from build123d import *

# Parameters (mm, degrees)
SKETCH_W        = 54.3
SKETCH_H        = 38
PAD_DEPTH       = 2
SKETCH001_W     = 54.3
SKETCH001_H     = 2
PAD001_DEPTH    = 22
SKETCH002_R     = 2.95
PAD002_DEPTH    = 5
SKETCH003_W     = 6.85
SKETCH003_H     = 15
PAD003_DEPTH    = 22
SKETCH004_R     = 1.5
POCKET_DEPTH    = 15
SKETCH005_W     = 6.85
SKETCH005_H     = 15
PAD004_DEPTH    = 22
SKETCH006_R     = 1.5
POCKET001_DEPTH = 15
CHAMFER_SIZE    = 0.5


with BuildPart() as part:
    # Sketch → Pad (new body)
    with BuildSketch(Plane.XY):
        with Locations((27.15, 21)):
            Rectangle(SKETCH_W, SKETCH_H)
    extrude(amount=PAD_DEPTH)

    # Sketch001 → Pad001 (join)
    with BuildSketch(Plane.XY):
        with Locations((27.15, 1)):
            Rectangle(SKETCH001_W, SKETCH001_H)
    extrude(amount=PAD001_DEPTH)

    # Sketch002 → Pad002 (join)
    with BuildSketch(Plane.XZ):
        with Locations((37.25, 12)):
            Circle(SKETCH002_R)
    extrude(amount=PAD002_DEPTH)

    # Sketch003 → Pad003 (join)
    with BuildSketch(Plane.XY):
        with Locations((3.425, 20.3)):
            Rectangle(SKETCH003_W, SKETCH003_H)
    extrude(amount=PAD003_DEPTH)

    # Sketch004 (on Face14 of Pad003) → Pocket (cut)
    with BuildSketch(Plane(origin=(0, 27.8, 0), x_dir=(-1, 0, 0), z_dir=(0, 1, 0))):
        with Locations((-3, 17)):
            Circle(SKETCH004_R)
        with Locations((-3, 7)):
            Circle(SKETCH004_R)
    extrude(amount=-POCKET_DEPTH, mode=Mode.SUBTRACT)

    # Sketch005 → Pad004 (join)
    with BuildSketch(Plane.XY):
        with Locations((50.875, 20.3)):
            Rectangle(SKETCH005_W, SKETCH005_H)
    extrude(amount=PAD004_DEPTH)

    # Sketch006 (on Face13 of Pad004) → Pocket001 (cut)
    with BuildSketch(Plane(origin=(0, 27.8, 0), x_dir=(-1, 0, 0), z_dir=(0, 1, 0))):
        with Locations((-51.3, 17)):
            Circle(SKETCH006_R)
        with Locations((-51.3, 7)):
            Circle(SKETCH006_R)
    extrude(amount=-POCKET001_DEPTH, mode=Mode.SUBTRACT)

    # Chamfer
    chamfer_edges = [part.edges().sort_by_distance(p)[0] for p in [
        (34.3, -5, 12),
    ]]
    chamfer(chamfer_edges, length=CHAMFER_SIZE)


solid = part.part
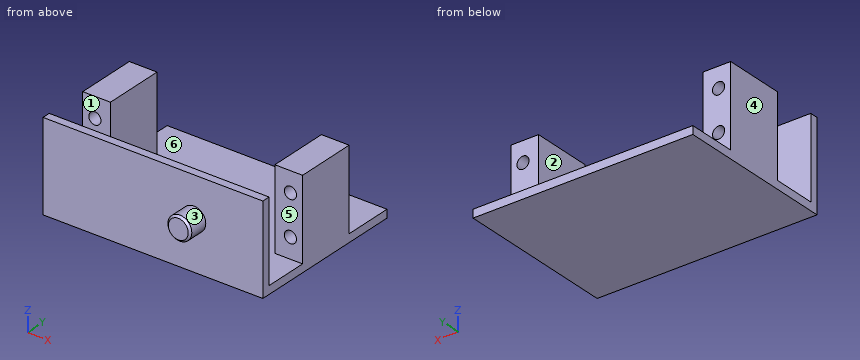
Could you check a few things on this model? Use its own coordinates, in mm. Face numbers are marked on the shaded views. A direction names the side the tool comes from. Round coordinates to 2 decimals unless told otherwise and drop trailing zeros. Write each loop counter-clockwise with the first axis right and the second up, starting at its lowest first coordinate (ties: lowest second). Pieces come first, ordered by that corner, then holes. Notation, with made-up numbers: (36.25, -40) - (45.25, -40) arc R26 ccw to (45.25, -24) - close; hole circle Ø9 at (18, 10.5). An arc over 180 degrees is marked (long way). Use a Markdown table: item, result.
Q1. I want a section at A-A (x = 51.3). List the corners of the cut face in (y, z) for me, plus the area to 3 significant figures.
Output values:
| item | result |
|---|---|
| outline | (0, 0) - (40, 0) - (40, 2) - (27.8, 2) - (27.8, 5.5) - (12.8, 5.5) - (12.8, 2) - (2, 2) - (2, 22) - (0, 22) - close; (12.8, 8.5) - (27.8, 8.5) - (27.8, 15.5) - (12.8, 15.5) - close; (12.8, 18.5) - (27.8, 18.5) - (27.8, 22) - (12.8, 22) - close |
| area | 330 mm2 |
Q2. For pin 1 (5 mm diameter, centred on x = 3, z = 7, fed in from -Y); pin 2 (5 mm diameter, centred on x = 46, y = 34, fed in from +Z); pin 3 (3.5 mm diameter, centred on x = 3, z = 17, fed in from +Y), each with a flat end and sliding along its axis, tell me the tip position at first contact or that it passes through.
Output values:
| item | result |
|---|---|
| pin 1 | y = 0 |
| pin 2 | z = 2 |
| pin 3 | y = 27.8 |
Q3. I want a section at B-B (z = 7). List the corners of the cut face in (x, y) for me.
Output values:
| item | result |
|---|---|
| outline | (0, 0) - (54.3, 0) - (54.3, 2) - (0, 2) - close; (0, 12.8) - (1.5, 12.8) - (1.5, 27.8) - (0, 27.8) - close; (4.5, 12.8) - (6.85, 12.8) - (6.85, 27.8) - (4.5, 27.8) - close; (47.45, 12.8) - (49.8, 12.8) - (49.8, 27.8) - (47.45, 27.8) - close; (52.8, 12.8) - (54.3, 12.8) - (54.3, 27.8) - (52.8, 27.8) - close |
Q4. Please list where these lines run through material, in increasing order: L1, parallel to Z at x = 3, y = 18; L2, parallel to X at y = 14.5, z = 9; L3, parallel to Y at x = 47.5, z = 14.5.
Output values:
| item | result |
|---|---|
| L1 | 0 to 5.5, 8.5 to 15.5, 18.5 to 22 |
| L2 | 0 to 6.85, 47.45 to 54.3 |
| L3 | 0 to 2, 12.8 to 27.8 |
Q5. For the marked faces 1, 2 and 3, which set-ups out of +Z, -Z, +X, -X, +Y, -Y let a thin tool reach every point of the face, with its end or its side?
Output values:
| item | result |
|---|---|
| face 1 | +Z, +X, -X |
| face 2 | +Z, +Y |
| face 3 | -Y |
Q6. I want a section at D-D (x = 33). List the corners of the cut face in (y, z) for me.
Output values:
| item | result |
|---|---|
| outline | (0, 0) - (40, 0) - (40, 2) - (2, 2) - (2, 22) - (0, 22) - close |
Q7. I want a section at C-C (z = 19.25). List the corners of the cut face in (x, y) for me.
Output values:
| item | result |
|---|---|
| outline | (0, 0) - (54.3, 0) - (54.3, 2) - (0, 2) - close; (0, 12.8) - (6.85, 12.8) - (6.85, 27.8) - (0, 27.8) - close; (47.45, 12.8) - (54.3, 12.8) - (54.3, 27.8) - (47.45, 27.8) - close |
Q8. Thinking about a two-plate mould opening in X: for the marked faces 4, 5 and 6, which applies, released by +X, released by -X, zero draft, split by the parting line, or undercut?
Output values:
| item | result |
|---|---|
| face 4 | released by -X |
| face 5 | zero draft |
| face 6 | undercut |
